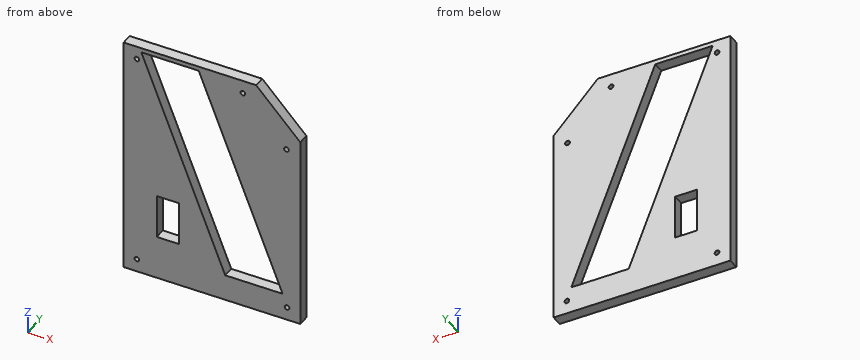
from build123d import *

# Parameters (mm, degrees)
SKETCH1_W               = 101.6
SKETCH1_H               = 139.7
BOSS_EXTRUDE1_DEPTH     = 6.35
CUT_EXTRUDE1_DEPTH      = 92.800885072
CUT_EXTRUDE4_DEPTH      = 92.800885072
CUT_EXTRUDE4_DEPTH_BACK = 6.35
CUT_EXTRUDE5_DEPTH      = 6.35
SKETCH11_W              = 12.7
SKETCH11_H              = 25.4
CUT_EXTRUDE6_DEPTH      = 6.35
SKETCH12_R              = 1.35255
CUT_EXTRUDE7_DEPTH      = 92.800885072


with BuildPart() as part:
    # Sketch1 → Boss-Extrude1 (new body)
    with BuildSketch(Plane(origin=(0, 0, 0), x_dir=(1, 0, 0), z_dir=(0, 1, 0))):
        with Locations((0, 6.35)):
            Rectangle(SKETCH1_W, SKETCH1_H)
    extrude(amount=BOSS_EXTRUDE1_DEPTH)

    # Sketch3 → Cut-Extrude1 (cut, through all)
    with BuildSketch(Plane(origin=(0, 6.35, 0), x_dir=(1, 0, 0), z_dir=(0, 1, 0))):
        with BuildLine():
            Line((-1.486564617, 31.962640907), (30.263435383, 59.140640907))
            ThreePointArc((30.263435383, 59.140640907), (33.486640907, 58.890564617), (33.236564617, 55.667359093))
            Line((33.236564617, 55.667359093), (1.486564617, 28.489359093))
            ThreePointArc((1.486564617, 28.489359093), (-1.736640907, 28.739435383), (-1.486564617, 31.962640907))
        make_face()
        with BuildLine():
            Line((1.486564617, -31.962640907), (-30.263435383, -59.140640907))
            ThreePointArc((-30.263435383, -59.140640907), (-33.486640907, -58.890564617), (-33.236564617, -55.667359093))
            Line((-33.236564617, -55.667359093), (-1.486564617, -28.489359093))
            ThreePointArc((-1.486564617, -28.489359093), (1.736640907, -28.739435383), (1.486564617, -31.962640907))
        make_face()
    extrude(amount=-CUT_EXTRUDE1_DEPTH, mode=Mode.SUBTRACT)

    # Sketch7 → Cut-Extrude4 (cut, two sides: drawn at the far end of the back side and taken through both)
    with BuildSketch(Plane(origin=(0, 6.35, 0), x_dir=(1, 0, 0), z_dir=(0, 1, 0)).offset(-CUT_EXTRUDE4_DEPTH_BACK)):
        Polygon((277.114298269, 200.961809181), (50.8, -36.813673481), (25.4, -63.5), (-200.914298269, -301.275482661), (274.636667054, -753.904079199), (752.665263592, -251.666787357), align=None)
    extrude(amount=CUT_EXTRUDE4_DEPTH + CUT_EXTRUDE4_DEPTH_BACK, mode=Mode.SUBTRACT)

    # Sketch10 → Cut-Extrude5 (cut)
    with BuildSketch(Plane(origin=(0, 6.35, 0), x_dir=(1, 0, 0), z_dir=(0, 1, 0))):
        Polygon((-40.64, -60.96), (-7.62, -60.96), (40.64, 60.96), (7.62, 60.96), align=None)
    extrude(amount=-CUT_EXTRUDE5_DEPTH, mode=Mode.SUBTRACT)

    # Sketch11 → Cut-Extrude6 (cut)
    with BuildSketch(Plane(origin=(0, 6.35, 0), x_dir=(1, 0, 0), z_dir=(0, 1, 0))):
        with Locations((-25.4, 38.1)):
            Rectangle(SKETCH11_W, SKETCH11_H)
    extrude(amount=-CUT_EXTRUDE6_DEPTH, mode=Mode.SUBTRACT)

    # Sketch12 → Cut-Extrude7 (cut, through all)
    with BuildSketch(Plane(origin=(0, 6.35, 0), x_dir=(1, 0, 0), z_dir=(0, 1, 0))):
        with Locations(Location((-43.18, 68.58, 0), (0, 0, 270))):
            Circle(SKETCH12_R)
        with Locations(Location((43.18, 68.58, 0), (0, 0, 90))):
            Circle(SKETCH12_R)
        with Locations(Location((-43.18, -55.88, 0), (0, 0, 90))):
            Circle(SKETCH12_R)
        with Locations(Location((17.78, -55.88, 0), (0, 0, 270))):
            Circle(SKETCH12_R)
        with Locations(Location((42.813150737, -29.579101009, 0), (0, 0, 90))):
            Circle(SKETCH12_R)
    extrude(amount=-CUT_EXTRUDE7_DEPTH, mode=Mode.SUBTRACT)


solid = part.part
The listing builds one solid part. Answer for the finished solid, in the listing's coordinates (mm). Round coordinates to 2 decimals unless told otherwise and drop trailing zeros. Order: outer loops, then holes, each group sorted by start corner. A loop starts at its lowest first (then second) coordinate and runs counter-clockwise, first axis right, second up. Notation, with made-up numbers: M 38.5,58 L 79.5,58 A16 ccw 79.5,76 Z; hole C 29.5,-8 d4. An arc over 180 degrees is marked long. Answer in a Markdown table with one row per item. Add a question column.
1) Consider line 1 along X through (y, z) = (3.25, -68.58); line 2 along Z through (x, y) = (-42.5, 3.5); line 3 along X through (y, z) = (2.25, 55.88). Determine where each line is inside the solid, lowest interval first. Write a range as from..to.
2) The part is cut by section C-C on y = 3. Determine the outline of the cut face in (x, z), plus the area to 3 significant figures.
3) The part is cut by section B-B on x = -38. Determine the outline of the cut face in (y, z).
4) Flat-ended cylindrical pins translate along their axes: pin 1 Ø2.5 at (x, z) = (-43.18, -68.58) entering from +Y; pin 2 Ø1 at (x, y) = (28.5, 5.5) entering from +Z. Find the tip coordinate at first contact, or state that the pin passes through.
5) The part is cut by section A-A on z = -31.5. Determine the outline of the cut face in (x, y), plus the area to 3 significant figures.
6) The part is cut by section D-D on z = 39. Determine the outline of the cut face in (x, y).
Findings below:
| question | item | result |
|---|---|---|
| 1 | line 1 | x = -50.8..-44.53, -41.83..41.83, 44.53..50.8 |
| 1 | line 2 | z = -76.2..-69.75, -67.41..54.71, 57.05..63.5 |
| 1 | line 3 | x = -50.8..-44.53, -41.83..-38.63, -5.61..16.43, 19.13..32.65 |
| 2 | outline | M -50.8,-76.2 L 50.8,-76.2 L 50.8,36.81 L 25.4,63.5 L -50.8,63.5 Z; hole C -43.18,-68.58 d2.71; hole C -43.18,55.88 d2.71; hole M -40.64,60.96 L 7.62,-60.96 L 40.64,-60.96 L -7.62,60.96 Z; hole M -31.75,-50.8 L -19.05,-50.8 L -19.05,-25.4 L -31.75,-25.4 Z; hole C 17.78,55.88 d2.71; hole C 42.81,29.58 d2.71; hole C 43.18,-68.58 d2.71 |
| 2 | area | 9,480 mm² |
| 3 | outline | M 0,-76.2 L 6.35,-76.2 L 6.35,54.29 L 0,54.29 Z; M 0,60.96 L 6.35,60.96 L 6.35,63.5 L 0,63.5 Z |
| 4 | pin 1 | passes through |
| 4 | pin 2 | stops at z = 60.77 |
| 5 | outline | M -50.8,0 L -31.75,0 L -31.75,6.35 L -50.8,6.35 Z; M -19.05,0 L -4.04,0 L -4.04,6.35 L -19.05,6.35 Z; M 28.98,0 L 50.8,0 L 50.8,6.35 L 28.98,6.35 Z |
| 5 | area | 355 mm² |
| 6 | outline | M -50.8,0 L -31.95,0 L -31.95,6.35 L -50.8,6.35 Z; M 1.07,0 L 48.72,0 L 48.72,6.35 L 1.07,6.35 Z |
